Input: part model. Units: mm. Frame: model coordinates. A direction names the side the tool comes from. Round coordinates to 2 decimals unless told otherwise and drop trailing zeros. Loops run counter-clockwise (first coordinate to the right, second up) from the corner with the lowest first, then second, coordinate; pieces in that order, holes last. Notation, with made-up numbers: (89, 62.5) -> (96, 62.5) arc R25 cw to (96, 94.5) -> close; hole circle Ø6 at (-37.75, 32.5). An arc over 180 degrees is marked (long way). Answer in a Markdown table with one row per item. Add a question column.
Q1. Pin query (flat end, axial travel): pin 1 (6 mm diameter, centred on x = 7.5, y = 8, fed in from -Z); pin 2 (4 mm diameter, centred on y = 8, z = 2.5, fed in from +X); pin 3 (5 mm diameter, centred on x = -11.5, z = 6, fed in from -Y); pin 4 (6 mm diameter, centred on x = -4, z = 6, fed in from +Y). Return the tip coordinate at first contact, or that it passes through.
Q2. Section A-A, the plane x = 0. Output: boundary loops of the cut face in (y, z), and give its area (3 significant figures).
Q3. Section D-D, the plane z = 3. Output: boundary loops of the cut face in (x, y).
Q4. Mould query, pull axis X, two halves, no side actions, for faces 3 (the face through (16, 12, 6.35)), 4 (the face through (-4.27, 0.56, 6.26)), 5 (the face through (-2.88, -21.91, 9.48)). Classes: pulls with the +X half, pulls with the -X half, needs draft (parallel to the pull), parting line crosses it, or undercut.
Q5. Reachability of faces 1 (the face through (14.62, 13.41, 3.13)), 2 (the face through (0, -5, 12.7)) from +Z, -Z, +X, -X, +Y, -Y: full face, straight path, thin tool, end or side. Return the list, or none.
Q6. Section C-C, the plane x = 15. Output: boundary loops of the cut face in (y, z).
Q7. Ray query, L1, parallel to Y at x = 0, z = 3.5; L2, parallel to Y at x = 0, z = 6.5; L3, parallel to X at y = -1, z = 11.75. Return the intervals inside material, ascending. Write a range as from..to.
Autodesk Inventor part; units mm, degrees
ref_plane "YZ Plane" through (0, 0, 0) normal (1, 0, 0) x (0, 1, 0)
ref_plane "XZ Plane" through (0, 0, 0) normal (0, 1, 0) x (-1, 0, 0)
ref_plane "XY Plane" through (0, 0, 0) normal (0, 0, 1) x (1, 0, 0)
sketch "Sketch1" plane through (0, 0, 0) normal (0, 0, 1) x (1, 0, 0)
  circle A0 centre (0, 0) radius 22.098
  dimension "d11" = 44.196
extrude "Extrusion1" add sketch "Sketch1" along normal blind 12.7
sketch "Sketch2" plane through (0, 0, 12.7) normal (0, 0, 1) x (1, 0, 0)
  circle A0 centre (0, 0) radius 22.098
hole "Hole1" at (0, 0, 12.7) direction (0, 0, -1) diameter 8.6106 depth 25.4 tip angle 118
sketch "Sketch3" plane through (0, 0, 0) normal (0, 0, -1) x (-1, 0, 0)
  circle A0 centre (0, 0) radius 4.3053
  circle A1 centre (0, 0) radius 22.098
sketch "Sketch4" plane through (0, 0, 0) normal (0, 0, -1) x (-1, 0, 0)
  circle A0 centre (0, 0) radius 22.098
  circle A1 centre (0, 0) radius 19.8374
  dimension "d12" = 39.6748
extrude "Extrusion2" cut sketch "Sketch4" against normal blind 6.35
thread "Thread1"
properties part number "JF-AT-TC0007" material "Acetal Resin, Black"
Answer block:
| question | item | result |
|---|---|---|
| 1 | pin 1 | z = 0 |
| 1 | pin 2 | x = 18.91 |
| 1 | pin 3 | y = -20.17 |
| 1 | pin 4 | y = 22.07 |
| 2 | outline | (-22.1, 6.35) -> (-19.84, 6.35) -> (-19.84, 0) -> (-4.31, 0) -> (-4.31, 12.7) -> (-22.1, 12.7) -> close; (4.31, 0) -> (19.84, 0) -> (19.84, 6.35) -> (22.1, 6.35) -> (22.1, 12.7) -> (4.31, 12.7) -> close |
| 2 | area | 423 mm^2 |
| 3 | outline | circle Ø39.67 at (0, 0); hole circle Ø8.61 at (0, 0) |
| 4 | face 3 | needs draft |
| 4 | face 4 | undercut |
| 4 | face 5 | parting line crosses it |
| 5 | face 1 | -Z |
| 5 | face 2 | +Z, +X, -X, +Y, -Y |
| 6 | outline | (-16.23, 6.35) -> (-12.98, 6.35) -> (-12.98, 0) -> (12.98, 0) -> (12.98, 6.35) -> (16.23, 6.35) -> (16.23, 12.7) -> (-16.23, 12.7) -> close |
| 7 | L1 | -19.84..-4.31, 4.31..19.84 |
| 7 | L2 | -22.1..-4.31, 4.31..22.1 |
| 7 | L3 | -22.08..-4.19, 4.19..22.08 |
